Can you work these out from the model? Positions are in its coordinate system, mm. Face numbers are marked on the shaded views. A direction names the side the tool comes from. Give positions to 0.01 mm unless a question says otherwise; leave off trailing zeros. Order: outer loops, then holes, each group sorted by start corner. A loop starts at its lowest first (then second) coordinate and runs counter-clockwise, first axis right, second up. Notation, with made-up numbers: (-24.5, 49) - (-12.5, 49) arc R21 ccw to (-12.5, 71) - close; hole circle Ø8 at (-35.75, 30). An arc over 180 degrees is marked (long way). One line per question, with ' | ' between items.
```python
from build123d import *

# Parameters (mm, degrees)
SKETCH1_W           = 54.102
SKETCH1_H           = 41.91
BOSS_EXTRUDE1_DEPTH = 1.5875
FILLET1_R           = 1.5875
SKETCH2_W           = 54.102
SKETCH2_H           = 25.4
BOSS_EXTRUDE2_DEPTH = 29.972
FILLET2_R           = 1.5875
FILLET3_R           = 1.5875
SKETCH3_RX          = 3.556
SKETCH3_RY          = 1.778
CUT_EXTRUDE1_DEPTH  = 2.5875
SKETCH4_W           = 9.906
SKETCH4_H           = 9.906
BOSS_EXTRUDE3_DEPTH = 11.43
CUT_EXTRUDE2_DEPTH  = 26.9080001


with BuildPart() as part:
    # Sketch1 → Boss-Extrude1 (new body)
    with BuildSketch(Plane.XY):
        Rectangle(SKETCH1_W, SKETCH1_H)
    extrude(amount=BOSS_EXTRUDE1_DEPTH)

    # Fillet1
    fillet1_edges = [part.edges().sort_by_distance(p)[0] for p in [
        (27.051, -20.955, 0.79375),
        (-27.051, -20.955, 0.79375),
        (-27.051, 20.955, 0.79375),
        (27.051, 20.955, 0.79375),
    ]]
    fillet(fillet1_edges, radius=FILLET1_R)

    # Sketch2 → Boss-Extrude2 (add)
    with BuildSketch(Plane(origin=(0, 0, 0), x_dir=(-1, 0, 0), z_dir=(0, 0, -1))):
        Rectangle(SKETCH2_W, SKETCH2_H)
    extrude(amount=BOSS_EXTRUDE2_DEPTH)

    # Fillet2
    fillet2_edges = [part.edges().sort_by_distance(p)[0] for p in [
        (0, 12.7, 0),
        (0, -12.7, 0),
    ]]
    fillet(fillet2_edges, radius=FILLET2_R)

    # Fillet3
    fillet3_edges = [part.edges().sort_by_distance(p)[0] for p in [
        (0, 12.7, -29.972),
        (0, -12.7, -29.972),
    ]]
    fillet(fillet3_edges, radius=FILLET3_R)

    # Sketch3 → Cut-Extrude1 (cut, through all)
    with BuildSketch(Plane(origin=(0, 0, 0), x_dir=(-1, 0, 0), z_dir=(0, 0, -1))):
        with Locations(Location((-12.065, -17.274273354), (0, 0, 180))):
            Ellipse(SKETCH3_RX, SKETCH3_RY)
        with Locations((12.065, -17.274273354)):
            Ellipse(SKETCH3_RX, SKETCH3_RY)
        with Locations((12.065, 17.274273354)):
            Ellipse(SKETCH3_RX, SKETCH3_RY)
        with Locations(Location((-12.065, 17.274273354), (0, 0, 180))):
            Ellipse(SKETCH3_RX, SKETCH3_RY)
    extrude(amount=-CUT_EXTRUDE1_DEPTH, mode=Mode.SUBTRACT)

    # Sketch4 → Boss-Extrude3 (add)
    with BuildSketch(Plane(origin=(27.051, 0, 0), x_dir=(0, 0, -1), z_dir=(1, 0, 0))):
        with Locations((14.097, 0)):
            Rectangle(SKETCH4_W, SKETCH4_H)
    extrude(amount=BOSS_EXTRUDE3_DEPTH)

    # Sketch6 → Cut-Extrude2 (cut, through all)
    with BuildSketch(Plane(origin=(0, 4.953, 0), x_dir=(1, 0, 0), z_dir=(0, 1, 0))):
        Polygon((38.481, 9.144), (28.575, 19.05), (38.481, 19.05), align=None)
    extrude(amount=-CUT_EXTRUDE2_DEPTH, mode=Mode.SUBTRACT)


solid = part.part
```
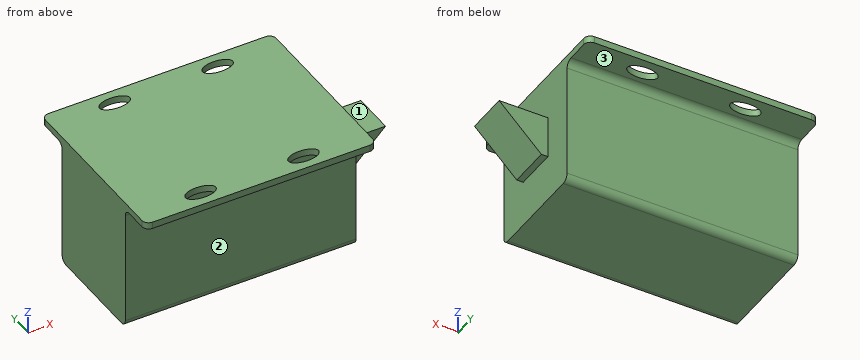
(1) On a 3-axis mill with a long thin cutter (end or side, diameter ignored), from which of +Z, -Z, +X, -X, +Y, -Y can I reach the whole of each face in a straight line? I mean the marked faces 1, 2 and 3. Say none if no direction works.
Answer below:
face 1: +Z, +X, +Y, -Y | face 2: -Z, +X, -X, -Y | face 3: -Z, +X, -X, +Y
(2) Imagine slicing it at B-B (z = -11.5). List the corners of the cut face in (x, y) for me (3 decimals), and give its area (3 significant figures).
Answer below:
outline: (-27.051, -12.7) - (27.051, -12.7) - (27.051, -4.953) - (36.125, -4.953) - (36.125, 4.953) - (27.051, 4.953) - (27.051, 12.7) - (-27.051, 12.7) - close | area: 1,460 mm^2
(3) Will these pins go through, and if not, where does the flat tip stop? pin 1 (10 mm diameter, centred on x = 8, z = -19, fed in from +Y); pin 2 (0.5 mm diameter, centred on x = 27.5, y = 0.5, fed in from -Z); pin 3 (12 mm diameter, centred on x = 28, y = -8, fed in from +Z); pin 4 (5 mm diameter, centred on x = 32, z = -12, fed in from +Y).
Answer below:
pin 1: y = 12.7 | pin 2: z = -19.05 | pin 3: z = 1.59 | pin 4: y = 4.95
(4) Imagine slicing it at D-D (x = 10.5). Count the separate pieces of the cut face and the enclosed holes in it, and give its area (3 significant figures).
Answer below:
separate pieces: 3 | enclosed holes: 0 | area: 818 mm^2
(5) Imagine slicing it at A-A (x = -21). List the corners of the cut face in (y, z) for me (1 decimal).
Answer below:
outline: (-21, 0) - (-14.3, 0) arc R1.6 cw to (-12.7, -1.6) - (-12.7, -28.4) arc R1.6 ccw to (-11.1, -30) - (11.1, -30) arc R1.6 ccw to (12.7, -28.4) - (12.7, -1.6) arc R1.6 cw to (14.3, 0) - (21, 0) - (21, 1.6) - (-21, 1.6) - close
(6) If I drill on line 1 (X direction, y = -7, z = -8); line 2 (Y direction, x = -8, z = -11); line 3 (Z direction, x = 21, y = -17.5), over which ranges is the centre line in solid material (lowest first)?
Answer below:
line 1: -27.05 to 27.05 | line 2: -12.7 to 12.7 | line 3: 0 to 1.59
